Check sheet for the modelled part. Datum: model origin and axes. Units: mm. A direction names the side the tool comes from. Round coordinates to 2 decimals unless told otherwise and drop trailing zeros. Order: outer loops, then holes, each group sorted by start corner. A loop starts at its lowest first (then second) coordinate and runs counter-clockwise, first axis right, second up. Notation, with made-up numbers: (-7.5, 7.25) -> (6.5, 7.25) arc R13 cw to (6.5, 27.25) -> close; hole circle Ø3 at (-7.5, 11). An arc over 180 degrees is marked (long way). Answer in a Markdown table with one row per item. Add a question column.
1. Depth check by flat-ended pin: P1, Ø1.7, axis at x = 38.5, y = 2, coming from the +Z side; P2, Ø5.5, axis at y = 1, z = -0.5, coming from the -X side; P3, Ø3, axis at x = 40.5, z = 7, coming from the -Y side. Enter the tip coordinate at first touch or a pass-through.
2. Draft check along Z on faces 5 (the flat face through (-1.016, -6, -2)), 6 (the cylindrical face through (0.5, -2.7, -2.9)), 7 (the cylindrical face through (-0.5, 8.07, -1.79)). Enter one of: +Z half, -Z half, draft (parallel to the pull), parting line (faces both ways), or undercut.
3. Sectioned sample at A-A, the plane x = 37.5. Record the boundary of the cut face in (y, z), then the cut area to 3 significant figures.
4. Material ranges on L1, parallel to Y at x = 0.3, z = 0; L2, parallel to Y at x = -0.3, z = 0; L3, parallel to X at y = -2.25, z = -4, recorded low to high. Write a range as from..to.
5. Access from +Z, -Z, +X, -X, +Y, -Y to the whole of each face (thin tool, end or side, straight path). Record for faces 1 (the flat face through (0, 4, 1)), 2 (the cylindrical face through (39.331, 8.738, -0.011)), 3 (the flat face through (39, 0, 7.938)), 4 (the flat face through (39, 0, -7.938)).
6. Sectioned sample at B-B, the plane x = 31.5. Record the boundary of the cut face in (y, z).
```python
from build123d import *

# Parameters (mm, degrees)
SKETCH1_W                 = 42.164
SKETCH1_H                 = 9.4361
SKETCH2_W                 = 1.016
SKETCH2_H                 = 3.9624
CUT_EXTRUDE1_DEPTH        = 5.588
SKETCH6_W                 = 10.8458
SKETCH6_H                 = 3.1623
FILLET1_R                 = 0.7874
F_8_32_TAPPED_HOLE1_D     = 3.4544
F_8_32_TAPPED_HOLE1_DEPTH = 10.668
F_8_32_TAPPED_HOLE1_TIP   = 1.037806461
SKETCH12_W                = 1.016
SKETCH12_H                = 2.5273


with BuildPart() as part:
    # Sketch1 → Revolve1 (revolve)
    with BuildSketch(Plane.XY, mode=Mode.PRIVATE) as revolve1_sk:
        with Locations((21.082, 4.71805)):
            Rectangle(SKETCH1_W, SKETCH1_H)
    revolve(revolve1_sk.sketch.rotate(Axis((-25.954653295, 0, 0), (1, 0, 0)), 90), axis=Axis((-25.954653295, 0, 0), (1, 0, 0)))  # turned: the seam where the file's is

    # Sketch2 → Cut-Revolve1 (revolve, cut)
    with BuildSketch(Plane.XY, mode=Mode.PRIVATE) as cut_revolve1_sk:
        with Locations((0.508, 1.9812)):
            Rectangle(SKETCH2_W, SKETCH2_H)
    revolve(cut_revolve1_sk.sketch.rotate(Axis((-4.423867111, 0, 0), (1, 0, 0)), 90), axis=Axis((-4.423867111, 0, 0), (1, 0, 0)), mode=Mode.SUBTRACT)  # turned: the seam where the file's is

    # Sketch3 → Cut-Revolve2 (revolve, cut)
    with BuildSketch(Plane.XY, mode=Mode.PRIVATE) as cut_revolve2_sk:
        Polygon((0, 8.3185), (5.1562, 8.3185), (6.2738, 9.4361), (0, 9.4361), align=None)
    revolve(cut_revolve2_sk.sketch.rotate(Axis((-2.146557548, 0, 0), (1, 0, 0)), 90), axis=Axis((-2.146557548, 0, 0), (1, 0, 0)), mode=Mode.SUBTRACT)  # turned: the seam where the file's is

    # Sketch4 → Cut-Revolve3 (revolve, cut)
    with BuildSketch(Plane.XY, mode=Mode.PRIVATE) as cut_revolve3_sk:
        Polygon((42.164, 8.7376), (36.576, 8.7376), (35.8775, 9.4361), (42.164, 9.4361), align=None)
    revolve(cut_revolve3_sk.sketch.rotate(Axis((-3.32735082, 0, 0), (1, 0, 0)), 90), axis=Axis((-3.32735082, 0, 0), (1, 0, 0)), mode=Mode.SUBTRACT)  # turned: the seam where the file's is

    # Sketch5 → Cut-Extrude1 (cut)
    with BuildSketch(Plane(origin=(42.164, 0, 0), x_dir=(0, 0, -1), z_dir=(1, 0, 0))):
        with BuildLine():
            Line((-7.9375, -3.652635694), (-7.9375, 0))
            Line((-7.9375, 0), (-7.9375, 3.652635694))
            ThreePointArc((-7.9375, 3.652635694), (-8.7376, 0), (-7.9375, -3.652635694))
        make_face()
        with BuildLine():
            Line((-3.96875004, 6.874076619), (-0.805474699, 8.700394489))
            ThreePointArc((-0.805474699, 8.700394489), (-4.3688, 7.566983568), (-7.132025301, 5.047758796))
            Line((-7.132025301, 5.047758796), (-3.96875004, 6.874076619))
        make_face()
        with BuildLine():
            ThreePointArc((7.132025301, 5.047758796), (4.3688, 7.566983568), (0.805474699, 8.700394489))
            Line((0.805474699, 8.700394489), (3.968749933, 6.874076681))
            Line((3.968749933, 6.874076681), (7.132025301, 5.047758796))
        make_face()
        with BuildLine():
            Line((7.9375, 3.652635694), (7.9375, 0))
            Line((7.9375, 0), (7.9375, -3.652635694))
            ThreePointArc((7.9375, -3.652635694), (8.535231507, -1.869619448), (8.7376, 0))
            ThreePointArc((8.7376, 0), (8.535231507, 1.869619448), (7.9375, 3.652635694))
        make_face()
        with BuildLine():
            Line((7.132025301, -5.047758796), (3.968749899, -6.874076701))
            Line((3.968749899, -6.874076701), (0.805474699, -8.700394489))
            ThreePointArc((0.805474699, -8.700394489), (4.3688, -7.566983568), (7.132025301, -5.047758796))
        make_face()
        with BuildLine():
            Line((-0.805474699, -8.700394489), (-3.96875004, -6.874076619))
            Line((-3.96875004, -6.874076619), (-7.132025301, -5.047758796))
            ThreePointArc((-7.132025301, -5.047758796), (-4.3688, -7.566983568), (-0.805474699, -8.700394489))
        make_face()
    extrude(amount=-CUT_EXTRUDE1_DEPTH, mode=Mode.SUBTRACT)

    # Sketch6 → Revolve3 (revolve)
    with BuildSketch(Plane.XY, mode=Mode.PRIVATE) as revolve3_sk:
        with Locations((47.5869, 1.58115)):
            Rectangle(SKETCH6_W, SKETCH6_H)
    revolve(revolve3_sk.sketch.rotate(Axis((-1.691095635, 0, 0), (1, 0, 0)), 90), axis=Axis((-1.691095635, 0, 0), (1, 0, 0)))  # turned: the seam where the file's is

    # Fillet1
    fillet1_edges = [part.edges().sort_by_distance(p)[0] for p in [
        (53.0098, 0, -3.1623),
    ]]
    fillet(fillet1_edges, radius=FILLET1_R)

    # #8-32 Tapped Hole1
    with Locations(Plane(origin=(53.0098, 0, 0), x_dir=(0, 0, -1), z_dir=(1, 0, 0))):
        with Locations((0, 0)):
            Hole(F_8_32_TAPPED_HOLE1_D / 2, depth=F_8_32_TAPPED_HOLE1_DEPTH)
            with Locations((0, 0, -(F_8_32_TAPPED_HOLE1_DEPTH + F_8_32_TAPPED_HOLE1_TIP / 2))):  # 118° drill point
                Cone(0, F_8_32_TAPPED_HOLE1_D / 2, F_8_32_TAPPED_HOLE1_TIP, mode=Mode.SUBTRACT)

    # Sketch12 → Revolve4 (revolve)
    with BuildSketch(Plane.XY, mode=Mode.PRIVATE) as revolve4_sk:
        with Locations((-0.508, 7.00405)):
            Rectangle(SKETCH12_W, SKETCH12_H)
    revolve(revolve4_sk.sketch.rotate(Axis((-4.807110581, 0, 0), (1, 0, 0)), 90), axis=Axis((-4.807110581, 0, 0), (1, 0, 0)))  # turned: the seam where the file's is


solid = part.part
```
Answer key:
| question | item | result |
|---|---|---|
| 1 | P1 | stops at z = 7.94 |
| 1 | P2 | stops at x = 1.02 |
| 1 | P3 | stops at y = -5.99 |
| 2 | face 5 | draft |
| 2 | face 6 | undercut |
| 2 | face 7 | parting line |
| 3 | outline | (-8.7, -0.81) -> (-5.05, -7.13) arc R8.74 ccw to (-3.65, -7.94) -> (3.65, -7.94) arc R8.74 ccw to (5.05, -7.13) -> (8.7, -0.81) arc R8.74 ccw to (8.7, 0.81) -> (5.05, 7.13) arc R8.74 ccw to (3.65, 7.94) -> (-3.65, 7.94) arc R8.74 ccw to (-5.05, 7.13) -> (-8.7, 0.81) arc R8.74 ccw to start |
| 3 | area | 216 mm² |
| 4 | L1 | y = -8.32..-3.96, 3.96..8.32 |
| 4 | L2 | y = -8.27..-5.74, 5.74..8.27 |
| 4 | L3 | x = 0..42.16 |
| 5 | face 1 | -X |
| 5 | face 2 | +X, +Y |
| 5 | face 3 | +Z, +X, +Y, -Y |
| 5 | face 4 | -Z, +X, +Y, -Y |
| 6 | outline | circle Ø18.87 at (0, 0) |
